Geometry: final body of the model. Coordinates: model frame, mm. Give positions to 0.01 mm unless a question says otherwise; leave off trailing zeros. Write each loop counter-clockwise with the first axis right and the second up, starting at its lowest first coordinate (ties: lowest second). Pieces come first, ordered by that corner, then holes.
Q1. Pin query (flat end, axial travel): pin 1 Ø1.5 at (x, z) = (8.5, 4.5) entering from -Y; pin 2 Ø1.9 at (y, z) = (29.5, 4) entering from -X; pin 3 Ø3 at (y, z) = (27, 1.5) entering from +X; pin 4 Ø4 at (x, y) = (0, -49.85) entering from +Z. Return the tip coordinate at first contact, or that it passes through.
Q2. Section A-A (x = 0). Return the cut outline in (y, z).
Q3. Line query: line 1 (Y direction, x = 0, z = 2); line 2 (X direction, y = -16.5, z = 5.5); line 3 (Y direction, x = 10.75, z = 1.5). Output: solid intervals per line, ascending.
Q4. Section C-C (x = 9). Return the cut outline in (y, z), plus the area to 3 significant figures.
Q5. Section D-D (y = 1). Return the cut outline in (x, z), plus the area to 3 significant figures.
Q6. Section B-B (z = 3.5). Return the cut outline in (x, y).
from build123d import *

# Parameters (mm, degrees)
CROQUIS1_R              = 3.5
SALIENTE_EXTRUIR1_DEPTH = 6.4


with BuildPart() as part:
    # Croquis1 → Saliente-Extruir1 (new body)
    with BuildSketch(Plane.XY):
        Polygon((-6, 15.149188933), (-6, -34.850811067), (-11.75, -44.850811067), (-11.75, -56.850811067), (-4.5, -64.850811067), (4.5, -64.850811067), (11.75, -56.850811067), (11.75, -44.850811067), (6, -34.850811067), (6, 15.149188933), (6, 65.149188933), (11.75, 75.149188933), (11.75, 87.149188933), (4.5, 95.149188933), (-4.5, 95.149188933), (-11.75, 87.149188933), (-11.75, 75.149188933), (-6, 65.149188933), align=None)
        with Locations((0, -49.850811067)):
            Circle(CROQUIS1_R, mode=Mode.SUBTRACT)
        with Locations((0, 80.149188933)):
            Circle(CROQUIS1_R, mode=Mode.SUBTRACT)
    extrude(amount=SALIENTE_EXTRUIR1_DEPTH)


solid = part.part
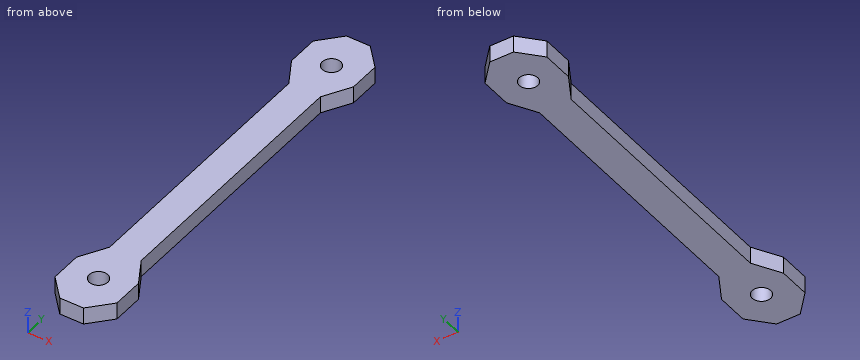
Computed:
1. pin 1: stops at y = -61.26
1. pin 2: stops at x = -6
1. pin 3: stops at x = 6
1. pin 4: passes through
2. outline: (-64.85, 0) - (-53.35, 0) - (-53.35, 6.4) - (-64.85, 6.4) - close; (-46.35, 0) - (76.65, 0) - (76.65, 6.4) - (-46.35, 6.4) - close; (83.65, 0) - (95.15, 0) - (95.15, 6.4) - (83.65, 6.4) - close
3. line 1: y = -64.85 to -53.35, -46.35 to 76.65, 83.65 to 95.15
3. line 2: x = -6 to 6
3. line 3: y = -57.95 to -43.11, 73.41 to 88.25
4. outline: (-59.89, 0) - (-40.07, 0) - (-40.07, 6.4) - (-59.89, 6.4) - close; (70.37, 0) - (90.18, 0) - (90.18, 6.4) - (70.37, 6.4) - close
4. area: 254 mm2
5. outline: (-6, 0) - (6, 0) - (6, 6.4) - (-6, 6.4) - close
5. area: 76.8 mm2
6. outline: (-11.75, -56.85) - (-4.5, -64.85) - (4.5, -64.85) - (11.75, -56.85) - (11.75, -44.85) - (6, -34.85) - (6, 65.15) - (11.75, 75.15) - (11.75, 87.15) - (4.5, 95.15) - (-4.5, 95.15) - (-11.75, 87.15) - (-11.75, 75.15) - (-6, 65.15) - (-6, -34.85) - (-11.75, -44.85) - close; hole circle Ø7 at (0, -49.85); hole circle Ø7 at (0, 80.15)
